Source: CAD feature listing. Evaluate the final solid. Frame: model axes, mm. A direction names the side the tool comes from. Round coordinates to 2 decimals unless told otherwise and drop trailing zeros. Loops run counter-clockwise (first coordinate to the right, second up) from the corner with the lowest first, then second, coordinate; pieces in that order, holes last.
Item 1: First-contact query: P1, Ø8, axis at x = 11.5, y = 13, coming from the +Z side. Flat tip, straight axial feed; report the tip coordinate or a pass-through.
Item 2: Section query C-C on z = 3.5. Return loops of the section in (x, y), then the cut area to 3 significant figures.
Item 3: Section query A-A on y = 39.5. Return loops of the section in (x, z).
Item 4: Pull-direction query (X, two-part tool) for faces 3 (the cylindrical face through (22.478, 0.362, 2.576)), 4 (the flat face through (4.844, 22.54, 3.828)), 5 (the flat face through (0, 23, 3)), 6 (the flat face through (18.052, 22.54, 3.792)); classes: released by +X, released by -X, zero draft, split by the parting line, or undercut.
Item 5: Section query D-D on x = 14. Return loops of the section in (y, z), then the cut area to 3 significant figures.
Item 6: Ray query, L1, parallel to Z at x = 12.5, y = 17.5; L2, parallel to X at y = 20.5, z = 3.7; L3, parallel to X at y = 32.5, z = 3.95. Return the intervals inside material, ascending.
Item 7: Section query B-B on x = 5. Return loops of the section in (y, z), then the cut area to 3 significant figures.
Item 8: Access query for faces 1 (the flat face through (11, 23, 2.54)), 2 (the cylindrical face through (0.362, 0.382, 2.576)). Directions: +Z, -Z, +X, -X, +Y, -Y. A direction counts if a zero-diameter tool reaches every point of the face in a straight line with its end or side. Return the directions, or none.
Autodesk Inventor part; units mm, degrees
ref_plane "YZ Plane" through (0, 0, 0) normal (1, 0, 0) x (0, 1, 0)
ref_plane "XZ Plane" through (0, 0, 0) normal (0, 1, 0) x (-1, 0, 0)
ref_plane "XY Plane" through (0, 0, 0) normal (0, 0, 1) x (1, 0, 0)
sketch "Sketch1" plane through (0, 0, 0) normal (0, 0, 1) x (1, 0, 0)
  line L0 (0, 0) -> (22.86, 0)
  line L1 (22.86, 0) -> (22.86, 45.72)
  line L2 (22.86, 45.72) -> (0, 45.72)
  line L3 (0, 45.72) -> (0, 0)
  dimension "d0" = 22.86
  dimension "d1" = 45.72
extrude "Extrusion1" add sketch "Sketch1" along normal blind 5.08
sketch "Sketch2" plane through (0, 0, 0) normal (0, -1, 0) x (1, 0, 0)
  line L0 (0, 5.08) -> (22.86, 5.08)
  line L1 (6.096, 5.08) -> (3.556, 2.54)
  line L2 (3.556, 2.54) -> (19.304, 2.54)
  line L3 (19.304, 2.54) -> (16.764, 5.08)
  line L4 (6.096, 5.08) -> (16.764, 5.08)
  line L5 (0, 0) -> (0, 5.08)
  line L6 (0, 0) -> (22.86, 0)
  dimension "d4" = 45
  dimension "d5" = 45
  dimension "d6" = 10.668
  dimension "d7" = 3.556
  dimension "d8" = 2.54
  dimension "d12" = 2.54
extrude "Extrusion2" cut sketch "Sketch2" against normal blind 50.8
fillet "Fillet1" radius 1.27 4 edges at (0, 0, 2.54) (22.86, 0, 2.54) (22.86, 45.72, 2.54) (0, 45.72, 2.54)
properties part number "nano_enclosure_modular_sidelock"
Data:
1. P1: stops at z = 2.54
2. outline: (0, 1.27) arc R1.27 ccw to (1.27, 0) - (4.52, 0) - (4.52, 45.72) - (1.27, 45.72) arc R1.27 ccw to (0, 44.45) - close; (18.34, 0) - (21.59, 0) arc R1.27 ccw to (22.86, 1.27) - (22.86, 44.45) arc R1.27 ccw to (21.59, 45.72) - (18.34, 45.72) - close
2. area: 412 mm2
3. outline: (0, 0) - (22.86, 0) - (22.86, 5.08) - (16.76, 5.08) - (19.3, 2.54) - (3.56, 2.54) - (6.1, 5.08) - (0, 5.08) - close
4. face 3: released by +X
4. face 4: undercut
4. face 5: released by -X
4. face 6: undercut
5. outline: (0, 0) - (45.72, 0) - (45.72, 2.54) - (0, 2.54) - close
5. area: 116 mm2
6. L1: z = 0 to 2.54
6. L2: x = 0 to 4.72, 18.14 to 22.86
6. L3: x = 0 to 4.97, 17.89 to 22.86
7. outline: (0, 0) - (45.72, 0) - (45.72, 2.54) - (0, 2.54) - close; (0, 3.98) - (45.72, 3.98) - (45.72, 5.08) - (0, 5.08) - close
7. area: 166 mm2
8. face 1: +Y, -Y
8. face 2: +Z, -Z, -X, -Y
